Could you check a few things on this model? Use its own coordinates, in mm. A direction names the side the tool comes from. Round coordinates to 2 decimals unless told otherwise and drop trailing zeros. Loops run counter-clockwise (first coordinate to the right, second up) from the corner with the lowest first, then second, coordinate; pieces in that order, holes last. Notation, with made-up numbers: (55, -8) - (100, -8) arc R9 ccw to (100, 6) - close; hole circle Ø1 at (14, 49.25). An arc over 180 degrees is marked (long way). Use one line per item in the form item = value.
```python
from build123d import *

# Parameters (mm, degrees)
BOSS_EXTRUDE1_DEPTH = 1.5
BOSS_EXTRUDE2_DEPTH = 1
FILLET1_R           = 0.5


with BuildPart() as part:
    # Sketch1 → Boss-Extrude1 (new body)
    with BuildSketch(Plane.XY):
        with BuildLine():
            Line((3.7329056464785526, 7.075691869668192), (3.032985837763823, 5.748999644105406))
            ThreePointArc((3.032985837763823, 5.748999644105406), (3.3567537930666855, -5.566166002980186), (-6.5, 0))
            Line((-6.5, 0), (-8, 9.8e-16))
            ThreePointArc((-8, 9.8e-16), (4.13138928377438, -6.850665849821768), (3.7329056464785526, 7.075691869668192))
        make_face()
    extrude(amount=BOSS_EXTRUDE1_DEPTH)

    # Sketch2 → Boss-Extrude2 (add)
    with BuildSketch(Plane.XY.offset(1.5)):
        with BuildLine():
            Line((3.7329056464785526, 7.075691869668192), (3.266292440668733, 6.191230385959669))
            ThreePointArc((3.266292440668733, 6.191230385959669), (3.6149656233025835, -5.994332618594048), (-7, 0))
            Line((-7, 0), (-8, 9.8e-16))
            ThreePointArc((-8, 9.8e-16), (4.13138928377438, -6.850665849821768), (3.7329056464785526, 7.075691869668192))
        make_face()
    extrude(amount=BOSS_EXTRUDE2_DEPTH)

    # Fillet1
    fillet1_edges = [part.edges().sort_by_distance(p)[0] for p in [
        (-6.5, -2.96e-15, 0.75),
        (-7, -3.17e-15, 2),
        (-8, 9.8e-16, 1.25),
        (3.2662924406687326, 6.191230385959669, 2),
        (3.032985837763823, 5.748999644105407, 0.75),
        (3.7329056464785557, 7.075691869668191, 1.25),
    ]]
    fillet(fillet1_edges, radius=FILLET1_R - 0.0001)  # a hair under: the kernel refuses the full size


solid = part.part
```
1. If we section it at C-C, the plane y = -2.75: Write out the boundary of the cut face in (x, z).
Solution:
outline = (-7.51, 0) - (-5.89, 0) - (-5.89, 1.5) - (-6.44, 1.5) - (-6.44, 2.5) - (-7.51, 2.5) - close; (5.89, 0) - (7.51, 0) - (7.51, 2.5) - (6.44, 2.5) - (6.44, 1.5) - (5.89, 1.5) - close
2. On a 3-axis mill with a long thin cutter (end or side, diameter ignored), from which of +Z, -Z, +X, -X, +Y, -Y can I reach the whole of each face in a straight line? I mean faces 1 (the face through (2.41, -6.21, 1.5)), 2 (the face through (3.51, -5.47, 0.74)). Say none if no direction works.
Solution:
face_1 = +Z
face_2 = +Z, -Z
3. If we section it at A-A, the plane x = 0: Write out the boundary of the cut face in (y, z), plus the area to 3 significant figures.
Solution:
outline = (-8, 0) - (-6.5, 0) - (-6.5, 1.5) - (-7, 1.5) - (-7, 2.5) - (-8, 2.5) - close
area = 3.25 mm^2
4. If we section it at D-D, the plane y = -4.75: Write out the boundary of the cut face in (x, z).
Solution:
outline = (-6.44, 0) - (-4.44, 0) - (-4.44, 1.5) - (-5.14, 1.5) - (-5.14, 2.5) - (-6.44, 2.5) - close; (4.44, 0) - (6.44, 0) - (6.44, 2.5) - (5.14, 2.5) - (5.14, 1.5) - (4.44, 1.5) - close
5. For P1, Ø1.5, axis at y = -2.5, z = 2, coming from the -X side; P2, Ø1, axis at x = 3.5, z = 1.5, coming from the -Y side, each with a flat end and sliding along its axis, tell me the tip position at first contact or that it passes through.
Solution:
P1 = -7.81
P2 = -7.42
6. If we section it at B-B, the plane z = 0.85: Write out the boundary of the cut face in (x, y).
Solution:
outline = (-7.98, -0.53) arc R8 ccw (long way) to (4.2, 6.81) arc R0.5 ccw to (3.49, 6.62) - (3.26, 6.18) arc R0.5 ccw to (3.44, 5.52) arc R6.5 cw (long way) to (-6.48, -0.46) arc R0.5 ccw to (-6.98, 0) - (-7.48, 0) arc R0.5 ccw to start
7. We'd pull the mould along Y, two halves only. Please class faces 3 (the face through (3, -7, 2.5)), 4 (the face through (3.93, -6.97, 1.23)), 5 (the face through (3.785, -5.888, 1.993)): +Y half, -Y half, draft (parallel to the pull), parting line (faces both ways), or undercut.
Solution:
face_3 = draft
face_4 = parting line
face_5 = undercut
8. Please list where these lines run through material, in increasing order: line 1 along Z through (x, y) = (-6, -3.5); line 2 along X through (y, z) = (-6, 2.05); line 3 along X through (y, z) = (-5.25, 2.25).
Solution:
line_1 = 0 to 1.5
line_2 = -5.29 to -3.61, 3.61 to 5.29
line_3 = -6.04 to -4.63, 4.63 to 6.04
